Design review of the part built by this model. Coordinates are the model's own, in mm. A direction names the side the tool comes from. Round coordinates to 2 decimals unless told otherwise and drop trailing zeros. Order: outer loops, then holes, each group sorted by start corner. A loop starts at its lowest first (then second) coordinate and runs counter-clockwise, first axis right, second up. Notation, with made-up numbers: (6.5, 38) - (17.5, 38) arc R7 ccw to (17.5, 51) - close; hole circle Ø3 at (83.25, -14). An arc over 180 degrees is marked (long way). Write item = value, one per line.
from build123d import *

# Parameters (mm, degrees)
BOSS_EXTRUDE1_DEPTH = 0.2
BOSS_EXTRUDE2_DEPTH = 12.58
SKETCH1_8_W         = 162.49
SKETCH1_8_H         = 1
BOSS_EXTRUDE3_DEPTH = 15.58
BOSS_EXTRUDE4_DEPTH = 12.38
BOSS_EXTRUDE5_DEPTH = 2.58


with BuildPart() as part:
    # Sketch1 → Boss-Extrude1 (new body)
    with BuildSketch(Plane(origin=(0, 0, 0), x_dir=(1, 0, 0), z_dir=(0, 1, 0))):
        Polygon((-113.845299462, 0), (-110.422649731, -5.92820323), (110.422649731, -5.92820323), (113.845299462, 0), (3.422649731, 191.25763964), (-3.422649731, 191.25763964), align=None)
        Polygon((108.979274058, -3.42820323), (-108.979274058, -3.42820323), (-110.958548116, 0), (-1.979274058, 188.75763964), (1.979274058, 188.75763964), (110.958548116, 0), align=None, mode=Mode.SUBTRACT)
    extrude(amount=BOSS_EXTRUDE1_DEPTH)

    # Sketch1_7 → Boss-Extrude2 (add)
    with BuildSketch(Plane(origin=(0, 0, 0), x_dir=(1, 0, 0), z_dir=(0, 1, 0))):
        Polygon((-95.137949192, 30.402081141), (-96.003974596, 30.902081141), (-113.845299462, 0), (-110.422649731, -5.92820323), (-74.74, -5.92820323), (-74.74, -4.92820323), (-109.845299462, -4.92820323), (-112.690598923, 0), align=None)
        Polygon((-3.422649731, 191.25763964), (-14.758974596, 171.622549002), (-13.892949192, 171.122549002), (-2.845299462, 190.25763964), (2.845299462, 190.25763964), (13.892949192, 171.122549002), (14.758974596, 171.622549002), (3.422649731, 191.25763964), align=None)
        Polygon((109.845299462, -4.92820323), (87.75, -4.92820323), (87.75, -5.92820323), (110.422649731, -5.92820323), (113.845299462, 0), (102.508974596, 19.635090638), (101.642949192, 19.135090638), (112.690598923, 0), align=None)
        Polygon((61.133974596, 91.298692801), (56.133974596, 99.958946839), (55.267949192, 99.458946839), (60.267949192, 90.798692801), align=None)
    extrude(amount=BOSS_EXTRUDE2_DEPTH)

    # Sketch1_8 → Boss-Extrude3 (add)
    with BuildSketch(Plane(origin=(0, 0, 0), x_dir=(1, 0, 0), z_dir=(0, 1, 0))):
        Polygon((-14.758974596, 171.622549002), (-96.003974596, 30.902081141), (-95.137949192, 30.402081141), (-13.892949192, 171.122549002), align=None)
        with Locations((6.505, -5.42820323)):
            Rectangle(SKETCH1_8_W, SKETCH1_8_H)
        Polygon((56.133974596, 99.958946839), (14.758974596, 171.622549002), (13.892949192, 171.122549002), (55.267949192, 99.458946839), align=None)
        Polygon((102.508974596, 19.635090638), (61.133974596, 91.298692801), (60.267949192, 90.798692801), (101.642949192, 19.135090638), align=None)
    extrude(amount=BOSS_EXTRUDE3_DEPTH)

    # Sketch1_9 → Boss-Extrude4 (add)
    with BuildSketch(Plane(origin=(0, 0, 0), x_dir=(1, 0, 0), z_dir=(0, 1, 0))):
        Polygon((-112.113248654, 0), (-110.834936491, -2.214101615), (-109.556624327, -4.42820323), (109.556624327, -4.42820323), (112.113248654, 0), (2.556624327, 189.75763964), (-2.556624327, 189.75763964), align=None)
        Polygon((-110.958548116, 0), (-56.468911087, 94.37881982), (-1.979274058, 188.75763964), (1.979274058, 188.75763964), (110.958548116, 0), (108.979274058, -3.42820323), (-108.979274058, -3.42820323), align=None, mode=Mode.SUBTRACT)
    extrude(amount=-BOSS_EXTRUDE4_DEPTH)

    # Sketch1_10 → Boss-Extrude5 (add)
    with BuildSketch(Plane(origin=(0, 0, 0), x_dir=(1, 0, 0), z_dir=(0, 1, 0))):
        Polygon((-95.137949192, 30.402081141), (-96.003974596, 30.902081141), (-113.845299462, 0), (-110.422649731, -5.92820323), (-74.74, -5.92820323), (-74.74, -4.92820323), (-109.845299462, -4.92820323), (-112.690598923, 0), align=None)
        Polygon((-3.422649731, 191.25763964), (-14.758974596, 171.622549002), (-13.892949192, 171.122549002), (-2.845299462, 190.25763964), (2.845299462, 190.25763964), (13.892949192, 171.122549002), (14.758974596, 171.622549002), (3.422649731, 191.25763964), align=None)
        Polygon((109.845299462, -4.92820323), (87.75, -4.92820323), (87.75, -5.92820323), (110.422649731, -5.92820323), (113.845299462, 0), (102.508974596, 19.635090638), (101.642949192, 19.135090638), (112.690598923, 0), align=None)
        Polygon((61.133974596, 91.298692801), (56.133974596, 99.958946839), (55.267949192, 99.458946839), (60.267949192, 90.798692801), align=None)
    extrude(amount=-BOSS_EXTRUDE5_DEPTH)


solid = part.part
Item 1: Take a section at A-A, the plane y = -6. State the section outline as (x, z) points, and give its area (3 significant figures).
Data:
outline = (-112.11, 0) - (-2.56, -189.76) - (2.56, -189.76) - (112.11, 0) - (109.56, 4.43) - (-109.56, 4.43) - close; hole (-110.96, 0) - (-1.98, -188.76) - (1.98, -188.76) - (110.96, 0) - (108.98, 3.43) - (-108.98, 3.43) - close
area = 669 mm2
Item 2: Insertion check: P1, Ø3, axis at y = 2, z = -41, coming from the +X side; P2, Ø0.8, axis at y = -1, z = 5.5, coming from the +X side; P3, Ø1.5, axis at x = 0.5, y = -6.5, coming from the -Z side; P4, Ø1.5, axis at x = -20.5, z = -154.5, coming from the +Y side. Each pin has a flat end and moves straight along its axis. Give the tip position at first contact, or say it passes through.
Data:
P1 = 91.04
P2 = 110.9
P3 = -189.76
P4 = through
Item 3: The part is to be moulded in two halves that separate along X. For faces 1 (the face through (112.11, 4.894, 3.006)), 2 (the face through (0, 6, -190.258)), 3 (the face through (35, 15.58, -136)), say which applies: +X half, -X half, draft (parallel to the pull), parting line (faces both ways), or undercut.
Data:
face_1 = +X half
face_2 = undercut
face_3 = draft
Item 4: Take a section at C-C, the plane x = 95. State the section outline as (y, z) points.
Data:
outline = (-12.38, -29.64) - (0, -29.64) - (0, -32.64) - (15.58, -32.64) - (15.58, -30.64) - (0.2, -30.64) - (0.2, -27.64) - (-12.38, -27.64) - close; (-12.38, 3.43) - (0.2, 3.43) - (0.2, 4.93) - (12.58, 4.93) - (12.58, 5.93) - (-2.58, 5.93) - (-2.58, 4.93) - (0, 4.93) - (0, 4.43) - (-12.38, 4.43) - close
Item 5: For faces 4 (the face through (-6, -2.58, -186)), 5 (the face through (-98.7, 12.58, 5.2)), 6 (the face through (57.733, -1.272, -95.189)), list the 3-axis set-ups (+Z, -Z, +X, -X, +Y, -Y) from which the entire face can be reached by the end or side of a thin tool; tool diameter is ignored.
Data:
face_4 = -Z, -Y
face_5 = +Z, -X, +Y
face_6 = -Y
Item 6: Take a section at B-B, the plane z = -12.5. State the section outline as (x, y) points, and give its area (3 significant figures).
Data:
outline = (-106.63, -2.58) - (-105.47, -2.58) - (-105.47, 0) - (-104.9, 0) - (-104.9, -12.38) - (-103.74, -12.38) - (-103.74, 0.2) - (-105.47, 0.2) - (-105.47, 12.58) - (-106.63, 12.58) - close; (103.74, -12.38) - (104.9, -12.38) - (104.9, 0) - (105.47, 0) - (105.47, -2.58) - (106.63, -2.58) - (106.63, 12.58) - (105.47, 12.58) - (105.47, 0.2) - (103.74, 0.2) - close
area = 64.3 mm2
Item 7: Take a section at D-D, the plane x = 40. State the section outline as (y, z) points, and give its area (3 significant figures).
Data:
outline = (-12.38, -124.9) - (0, -124.9) - (0, -127.9) - (15.58, -127.9) - (15.58, -125.9) - (0.2, -125.9) - (0.2, -122.9) - (-12.38, -122.9) - close; (-12.38, 3.43) - (0.2, 3.43) - (0.2, 4.93) - (15.58, 4.93) - (15.58, 5.93) - (0, 5.93) - (0, 4.43) - (-12.38, 4.43) - close
area = 84.8 mm2
Item 8: For line 1 along Z through (x, y) = (-52.5, 2.5); line 2 along Z through (x, y) = (94, 3.25); line 3 along X through (y, z) = (7.75, -170.5), list the stretches that pass through material, from the lowest coordinate up. Write a range as [from, to].
Data:
line_1 = [-106.25, -104.25], [4.93, 5.93]
line_2 = [-34.37, -32.37], [4.93, 5.93]
line_3 = [-15.41, -14.25], [14.25, 15.41]
